```python
from build123d import *

# Parameters (mm, degrees)
SKETCH_1_W                     = 12
SKETCH_1_H                     = 80
EXTRUDE_1_DEPTH                = 8
SKETCH_2_R                     = 3
CUT_EXTRUDE_1_DEPTH            = 5
HOLE_WIZARD_M2_5_1_D           = 2.9
HOLE_WIZARD_M2_5_1_CSINK_D     = 5.5
HOLE_WIZARD_M2_5_1_CSINK_ANGLE = 90
HOLE_WIZARD_M2_5_2_D           = 2.9
HOLE_WIZARD_M2_5_2_CSINK_D     = 5.5
HOLE_WIZARD_M2_5_2_CSINK_ANGLE = 90
F_1_0MM_2_REACH                = 44.521
F_1_0MM_2_BORE_R               = 1.35


with BuildPart() as part:
    # 草圖1 → 填料-伸長1 (new body)
    with BuildSketch(Plane(origin=(0, 0, 0), x_dir=(0, 0, -1), z_dir=(1, 0, 0))):
        Rectangle(SKETCH_1_W, SKETCH_1_H)
    extrude(amount=EXTRUDE_1_DEPTH)

    # 草圖2 → 除料-伸長1 (cut)
    with BuildSketch(Plane.ZY):
        with Locations((0, -35)):
            Circle(SKETCH_2_R)
    extrude(amount=-CUT_EXTRUDE_1_DEPTH, mode=Mode.SUBTRACT)

    # M2.5 錐坑平頭螺釘的錐孔1 (through all)
    with Locations(Plane(origin=(8, 0, 0), x_dir=(0, 0, -1), z_dir=(1, 0, 0))):
        with Locations((0, -35)):
            CounterSinkHole(HOLE_WIZARD_M2_5_1_D / 2, HOLE_WIZARD_M2_5_1_CSINK_D / 2, counter_sink_angle=HOLE_WIZARD_M2_5_1_CSINK_ANGLE)

    # M2.5 錐坑平頭螺釘的錐孔2 (through all)
    with Locations(Plane.ZY):
        with Locations((0, 36.5), (0, 28.5)):
            CounterSinkHole(HOLE_WIZARD_M2_5_2_D / 2, HOLE_WIZARD_M2_5_2_CSINK_D / 2, counter_sink_angle=HOLE_WIZARD_M2_5_2_CSINK_ANGLE)

    # Ø1.0mm 定位孔2 bore → Ø1.0mm 定位孔2 (cut, up to next)
    with BuildSketch(Plane.XY.offset(6), mode=Mode.PRIVATE) as f_1_0mm_2_sk1:
        with Locations((3, -35)):
            Circle(F_1_0MM_2_BORE_R)
    f_1_0mm_2_tool1 = extrude(f_1_0mm_2_sk1.sketch, amount=-F_1_0MM_2_REACH, mode=Mode.PRIVATE) & part.part
    f_1_0mm_2 = f_1_0mm_2_tool1.solids().sort_by_distance((3, -35, 6))[0]
    add(f_1_0mm_2, mode=Mode.SUBTRACT)

    # 鏡射1: Ø1.0mm 定位孔2 across plane
    add(f_1_0mm_2.mirror(Plane.XY), mode=Mode.SUBTRACT)


solid = part.part
```
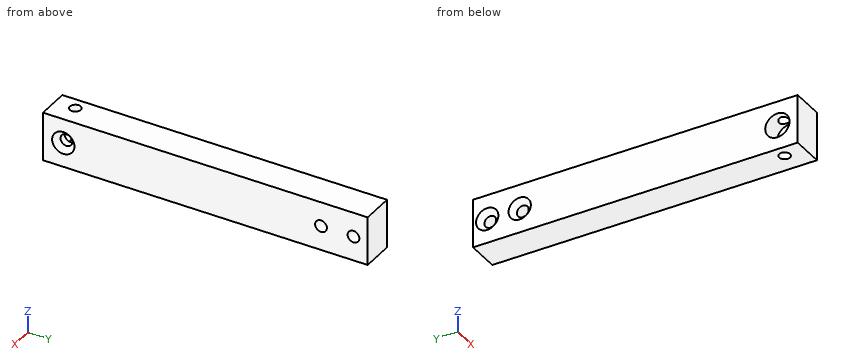
Build history of the part. All positions in model axes, mm. Give positions to 0.01 mm unless a question says otherwise; leave off trailing zeros. Loops run counter-clockwise (first coordinate to the right, second up) from the corner with the lowest first, then second, coordinate; pieces in that order, holes last.
1) Probe line 1 along Y through (x, z) = (3.3, 0); line 2 along Y through (x, z) = (3, -4.95); line 3 along Z through (x, y) = (5, 36.5). List the from-to ranges inside material, lowest first.
Values follow:
line 1: y = -40 to -38, -32 to 27.05, 29.95 to 35.05, 37.95 to 40
line 2: y = -40 to -36.35, -33.65 to 40
line 3: z = -6 to -1.45, 1.45 to 6
2) Band-saw the part on C-C on y = 36.5. List the corners of the cut face in (x, z).
Values follow:
outline: (0, -6) - (8, -6) - (8, -1.45) - (1.3, -1.45) - (0, -2.75) - close; (0, 2.75) - (1.3, 1.45) - (8, 1.45) - (8, 6) - (0, 6) - close
3) Band-saw the part on A-A on x = 3. List the corners of the cut face in (y, z).
Values follow:
outline: (-40, -6) - (-36.35, -6) - (-36.35, -2.68) arc R3 cw to (-36.35, 2.68) - (-36.35, 6) - (-40, 6) - close; (-33.65, -6) - (40, -6) - (40, 6) - (-33.65, 6) - (-33.65, 2.68) arc R3 cw to (-33.65, -2.68) - close; hole circle Ø2.9 at (28.5, 0); hole circle Ø2.9 at (36.5, 0)
4) Band-saw the part on B-B on y = -35. List the corners of the cut face in (x, z).
Values follow:
outline: (0, -6) - (1.65, -6) - (1.65, -3) - (0, -3) - close; (0, 3) - (1.65, 3) - (1.65, 6) - (0, 6) - close; (4.35, -6) - (8, -6) - (8, -2.75) - (6.7, -1.45) - (5, -1.45) - (5, -3) - (4.35, -3) - close; (4.35, 3) - (5, 3) - (5, 1.45) - (6.7, 1.45) - (8, 2.75) - (8, 6) - (4.35, 6) - close
